```python
from build123d import *

# Parameters (mm, degrees)
BOSS_EXTRUDE1_DEPTH = 2
SKETCH2_R           = 1.5
SKETCH2_R_2         = 3
CUT_EXTRUDE1_DEPTH  = 2


with BuildPart() as part:
    # Sketch1 → Boss-Extrude1 (new body)
    with BuildSketch(Plane.XY):
        Polygon((0, -15), (0, 0), (204, 0), (204, -15), (152, -15), (152, -13), (52, -13), (52, -15), align=None)
    boss_extrude1 = extrude(amount=BOSS_EXTRUDE1_DEPTH)

    # Mirror2: Boss-Extrude1 across plane
    add(boss_extrude1.mirror(Plane(origin=(0, 0, 2), x_dir=(0, 0, 1), z_dir=(0, -1, 0))))

    # Sketch2 → Cut-Extrude1 (cut)
    with BuildSketch(Plane.XY.offset(2)):
        with Locations((6.5, 0)):
            Circle(SKETCH2_R)
        with Locations((15, 0)):
            Circle(SKETCH2_R_2)
        with Locations((23.5, 0)):
            Circle(SKETCH2_R)
        with Locations((180.5, 0)):
            Circle(SKETCH2_R)
        with Locations((189, 0)):
            Circle(SKETCH2_R_2)
        with Locations((197.5, 0)):
            Circle(SKETCH2_R)
    extrude(amount=-CUT_EXTRUDE1_DEPTH, mode=Mode.SUBTRACT)


solid = part.part
```
The model under review builds one solid part; all positions refer to its coordinate system, in mm. Round coordinates to 2 decimals unless told otherwise and drop trailing zeros. Order: outer loops, then holes, each group sorted by start corner. A loop starts at its lowest first (then second) coordinate and runs counter-clockwise, first axis right, second up. Notation, with made-up numbers: (48, 64.5) -> (72, 64.5) arc R22 ccw to (72, 77.5) -> close; hole circle Ø8 at (43, 52). An arc over 180 degrees is marked (long way). One line per item, written item: value. Start each with the question number.
Q1. Take a section at C-C (x = 147.5). Write out the cut boundary in (y, z).
Q2. Take a section at A-A (x = 189). Write out the cut boundary in (y, z), and give its area (3 significant figures).
Q3. Clearance check with a flat-ended pin moving along its axis: pin 1 Ø1 at (x, z) = (79, 0.5) entering from +Y. State where the tip first meets the part, or that it passes through.
Q4. Take a section at B-B (z = 0.7). Write out the cut boundary in (x, y).
Q5. Mouldability with a two-part tool opening along X and no side actions: class faces 1 (the face through (103, 0, 0)), 2 (the face through (191.86, 0.9, 1.01)) as released by +X, released by -X, zero draft, split by the parting line, or undercut.
Q6. Wall thickness on line 1 (Y direction, x = 15, z = 1.3); line 2 (X direction, y = 1.75, z = 1.6); line 3 (Y direction, x = 23.5, z = 0.9): over which ranges is each line inside the solid? List them lowest first.
Reported:
1. outline: (-13, 0) -> (13, 0) -> (13, 2) -> (-13, 2) -> close
2. outline: (-15, 0) -> (-3, 0) -> (-3, 2) -> (-15, 2) -> close; (3, 0) -> (15, 0) -> (15, 2) -> (3, 2) -> close
2. area: 48.0 mm2
3. pin 1: stops at y = 13
4. outline: (0, -15) -> (52, -15) -> (52, -13) -> (152, -13) -> (152, -15) -> (204, -15) -> (204, 15) -> (152, 15) -> (152, 13) -> (52, 13) -> (52, 15) -> (0, 15) -> close; hole circle Ø3 at (6.5, 0); hole circle Ø6 at (15, 0); hole circle Ø3 at (23.5, 0); hole circle Ø3 at (180.5, 0); hole circle Ø6 at (189, 0); hole circle Ø3 at (197.5, 0)
5. face 1: zero draft
5. face 2: undercut
6. line 1: y = -15 to -3, 3 to 15
6. line 2: x = 0 to 12.56, 17.44 to 186.56, 191.44 to 204
6. line 3: y = -15 to -1.5, 1.5 to 15
